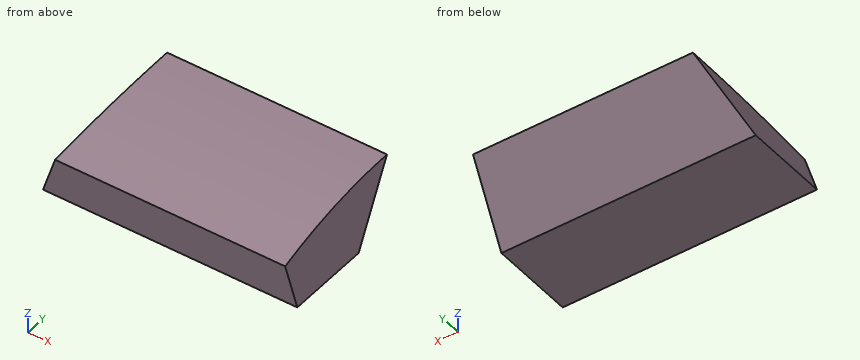
```python
from build123d import *

# Parameters (mm, degrees)
F1_DEPTH = 609.6
F3_DEPTH = 709.1064125189


with BuildPart() as f1:
    # F0 (on Right) → F1 (new body)
    with BuildSketch(Plane.YZ):
        with BuildLine():
            Line((-406.4, 179.4700178945), (-406.4, 0))
            Line((-406.4, 0), (0, 0))
            Line((0, 0), (302.7054125189, 254))
            ThreePointArc((302.7054125189, 254), (-53.8002691666, 235.3163289211), (-406.4, 179.4700178945))
        make_face()
    extrude(amount=F1_DEPTH)

    # F2 (on face) → F3 (cut, through all)
    with BuildSketch(Plane.XZ.offset(406.4)):
        Polygon((551.2866563028, 179.4700178945), (609.6, 0), (609.6, 179.4700178945), align=None)
        Polygon((519.0783191877, 278.5970867934), (551.2866563028, 179.4700178945), (609.6, 179.4700178945), (609.6, 278.5970867934), align=None)
    extrude(amount=-F3_DEPTH, mode=Mode.SUBTRACT)

    # F4: F1 across plane


with BuildPart() as f1_1:
    add(f1.part)
    add(f1.part.mirror(Plane.YZ))


solid = f1_1.part
```
Here's how the part is built. I have some questions about the finished solid (model axes, mm). Coordinates: 2 decimals unless noted, no trailing zeros. Write each loop counter-clockwise with the first axis right and the second up, starting at its lowest first coordinate (ties: lowest second). Pieces come first, ordered by that corner, then holes. Notation, with made-up numbers: M 2.5,31.5 L 45.5,31.5 A34 ccw 45.5,69.5 Z; hole C 60,7 d9. An arc over 180 degrees is marked long. Answer as CSV lines item,"result". Start each with the question number.
Q1. Will these pins go through, and if not, where does the flat tip stop? pin 1 Ø12 at (y, z) = (17, 75) entering from +X; pin 2 Ø1 at (y, z) = (-47, 188.5) entering from +X; pin 3 Ø1.5 at (x, z) = (353.5, 102.5) entering from +Y; pin 4 Ø10 at (x, y) = (63, -209.5) entering from -Z.
Q2. I need wall thicknesses on probe 1 along X at (y, z) = (-251, 91); probe 2 along Y at (x, z) = (-438, 168); probe 3 along X at (y, z) = (60, 81). Which ranges of each line are inside material? Lowest first, please. Write a range as [from, to].
Q3. Suppose I cut it at B-B, the plane y = -139.5. List the corners of the cut face in (x, z) for me, then the cut area to 3 significant figures.
Q4. Suppose I cut it at A-A, the plane x = 349.5. List the corners of the cut face in (y, z) for me.
Entries:
1,pin 1,"stops at x = 587.18"
1,pin 2,"stops at x = 548.52"
1,pin 3,"stops at y = 123.05"
1,pin 4,"stops at z = 0"
2,probe 1,"x = [-580.03, 580.03]"
2,probe 2,"y = [-406.4, 200.21]"
2,probe 3,"x = [-583.28, 583.28]"
3,outline,"M -609.6,0 L 609.6,0 L 536.42,225.21 L -536.42,225.21 Z"
3,area,"258,000 mm²"
4,outline,"M -406.4,0 L 0,0 L 302.71,254 A3410.61 ccw -406.4,179.47 Z"
